Model file for the job. Use its own axes, mm. A direction names the side the tool comes from. Coordinates: 2 decimals unless noted, no trailing zeros. Write each loop counter-clockwise with the first axis right and the second up, starting at its lowest first coordinate (ties: lowest second). Pieces come first, ordered by that corner, then holes. Notation, with made-up numbers: M 67.5,84 L 101.5,84 A30 cw 101.5,106 Z; hole C 49.25,84 d9. An arc over 180 degrees is marked long. One line per question, with ' | ' between items. Start each with the question number.
(1) Cut at A-A (y = 17.5). Write the cut outline in (x, z), plus the area to 3 significant figures.
(2) Two-plate mould, pull along Z, no slides. Class faces 3 (the face through (-2.8, -25, 17.9)), 4 (the face through (-4, -2.5, 18)), 5 (the face through (0, 0, 0)): +Z half, -Z half, draft (parallel to the pull), parting line (faces both ways), or undercut.
(3) Flat gauge pins, fed straight in: pin 1 Ø2.5 at (x, y) = (10, -17.5) entering from -Z; pin 2 Ø5 at (x, y) = (0, -7.45) entering from +Z. Where does each tip first touch, or does it go through?
(4) Cut at D-D (x = 3). Write the cut outline in (y, z), plus the area to 3 significant figures.
(5) Cut at B-B (z = 13.4). Write the cut outline in (x, y).
(6) Wall check: probe 1 along Y at (x, z) = (-10.25, 6.25); probe 2 along Y at (x, z) = (0, 0.85); probe 3 along Z at (x, y) = (0, -25.9). Give the ranges that are in metal, low to high.
(7) Tool access for faces 1 (the face through (15, 0, 9)), 2 (the face through (0, 13, 4)): list every direction of +Z, -Z, +X, -X, +Y, -Y with a clear straight run to the whole face (end or side of a thin tool).
(8) Cut at C-C (x = -10). Write the cut outline in (y, z).
from build123d import *

# Parameters (mm, degrees)
F0_W     = 30
F0_H     = 55
F1_DEPTH = 4
F2_R     = 2
F3_DEPTH = 4
F4_W     = 30
F4_H     = 5
F5_DEPTH = 20
F6_R     = 5.3
F7_DEPTH = 55.001
F8_R     = 2
F9_DEPTH = 4


with BuildPart() as f1:
    # F0 (on Top) → F1 (new body)
    with BuildSketch(Plane.XY):
        Rectangle(F0_W, F0_H)
    extrude(amount=F1_DEPTH)

    # F2 (on face) → F3 (cut)
    with BuildSketch(Plane.XY.offset(4)):
        with Locations((0, -17.5)):
            Circle(F2_R)
        with Locations((0, 17.5)):
            Circle(F2_R)
    extrude(amount=-F3_DEPTH, mode=Mode.SUBTRACT)

    # F4 (on face) → F5 (join)
    with BuildSketch(Plane.XY.offset(4)):
        with Locations((0, 25)):
            Rectangle(F4_W, F4_H)
        Rectangle(F4_W, F4_H)
        with Locations((0, -25)):
            Rectangle(F4_W, F4_H)
    extrude(amount=F5_DEPTH)

    # F6 (on face) → F7 (cut, through all)
    with BuildSketch(Plane(origin=(0, 27.5, 0), x_dir=(-1, 0, 0), z_dir=(0, 1, 0))):
        with Locations((0, 13.4)):
            Circle(F6_R)
    extrude(amount=-F7_DEPTH, mode=Mode.SUBTRACT)

    # F8 (on face) → F9 (cut)
    with BuildSketch(Plane(origin=(0, 0, 0), x_dir=(1, 0, 0), z_dir=(0, 0, -1))):
        with Locations((10, -17.5)):
            Circle(F8_R)
        with Locations((10, -7.446962)):
            Circle(F8_R)
        with Locations((-10, -17.5)):
            Circle(F8_R)
        with Locations((-10, -7.446962)):
            Circle(F8_R)
        with Locations((-10, 7.446962)):
            Circle(F8_R)
        with Locations((-10, 17.5)):
            Circle(F8_R)
        with Locations((10, 17.5)):
            Circle(F8_R)
        with Locations((10, 7.446962)):
            Circle(F8_R)
        with Locations((0, -7.446962)):
            Circle(F8_R)
        with Locations((0, 7.446962)):
            Circle(F8_R)
    extrude(amount=-F9_DEPTH, mode=Mode.SUBTRACT)


solid = f1.part
Filled in:
1) outline: M -15,0 L -12,0 L -12,4 L -15,4 Z; M -8,0 L -2,0 L -2,4 L -8,4 Z; M 2,0 L 8,0 L 8,4 L 2,4 Z; M 12,0 L 15,0 L 15,4 L 12,4 Z | area: 72.0 mm²
2) face 3: undercut | face 4: draft | face 5: -Z half
3) pin 1: through | pin 2: z = 4
4) outline: M -27.5,0 L 27.5,0 L 27.5,9.03 L 22.5,9.03 L 22.5,4 L 2.5,4 L 2.5,9.03 L -2.5,9.03 L -2.5,4 L -22.5,4 L -22.5,9.03 L -27.5,9.03 Z; M -27.5,17.77 L -22.5,17.77 L -22.5,24 L -27.5,24 Z; M -2.5,17.77 L 2.5,17.77 L 2.5,24 L -2.5,24 Z; M 22.5,17.77 L 27.5,17.77 L 27.5,24 L 22.5,24 Z | area: 389 mm²
5) outline: M -15,-27.5 L -5.3,-27.5 L -5.3,-22.5 L -15,-22.5 Z; M -15,-2.5 L -5.3,-2.5 L -5.3,2.5 L -15,2.5 Z; M -15,22.5 L -5.3,22.5 L -5.3,27.5 L -15,27.5 Z; M 5.3,-27.5 L 15,-27.5 L 15,-22.5 L 5.3,-22.5 Z; M 5.3,-2.5 L 15,-2.5 L 15,2.5 L 5.3,2.5 Z; M 5.3,22.5 L 15,22.5 L 15,27.5 L 5.3,27.5 Z
6) probe 1: -27.5 to -22.5, -2.5 to 2.5, 22.5 to 27.5 | probe 2: -27.5 to -19.5, -15.5 to -9.45, -5.45 to 5.45, 9.45 to 15.5, 19.5 to 27.5 | probe 3: 0 to 8.1, 18.7 to 24
7) face 1: +Z, -Z, +X, +Y, -Y | face 2: +Z, +X, -X
8) outline: M -27.5,0 L -19.5,0 L -19.5,4 L -22.5,4 L -22.5,24 L -27.5,24 Z; M -15.5,0 L -9.45,0 L -9.45,4 L -15.5,4 Z; M -5.45,0 L 5.45,0 L 5.45,4 L 2.5,4 L 2.5,24 L -2.5,24 L -2.5,4 L -5.45,4 Z; M 9.45,0 L 15.5,0 L 15.5,4 L 9.45,4 Z; M 19.5,0 L 27.5,0 L 27.5,24 L 22.5,24 L 22.5,4 L 19.5,4 Z
